Check sheet for the modelled part. Datum: model origin and axes. Units: mm. Face numbers are marked on the shaded views. A direction names the side the tool comes from. Give positions to 0.01 mm unless a question says otherwise; leave off trailing zeros. Loops run counter-clockwise (first coordinate to the right, second up) from the corner with the lowest first, then second, coordinate; pieces in that order, holes last. Notation, with made-up numbers: (8.25, 7.25) -> (20.25, 7.25) arc R17 cw to (20.25, 13.25) -> close; hole circle Ø3 at (85, -25.75). An arc over 180 degrees is marked (long way). Answer as CSV lines item,"result". Start each with the question number.
(1) Gauge pin test, flat end, axial feed: pin 1 Ø0.6 at (x, z) = (15, 1) entering from -Y. Record the tip position at first contact, or that the pin passes through.
(2) Material ranges on line 1 (Y direction, x = 13.45, z = 1.35) (3 decimals); line 2 (X direction, y = 2.5, z = 1.25); line 3 (Y direction, x = 2, z = 1) (3 decimals), recorded low to high. Write a range as from..to.
(3) Section check B-B on z = 1.45. Enter the section's corners in (x, y) (3 decimals), plus the area to 3 significant figures.
(4) Section check C-C on x = 1.5. Enter the section's corners in (y, z) (1 decimal).
(5) Release check for a two-part mould opening along Y. For the marked faces 4, 5, 6 and 7 record: pulls with the +Y half, pulls with the -Y half, needs draft (parallel to the pull), parting line crosses it, or undercut.
(6) Access from +Z, -Z, +X, -X, +Y, -Y to the whole of each face (thin tool, end or side, straight path). Record for the marked faces 1, 2 and 3.
(7) Section check A-A on x = 13.45. Enter the section's corners in (y, z) (3 decimals), plus the area to 3 significant figures.
from build123d import *

# Parameters (mm, degrees)
SKETCH2_R           = 0.95
BOSS_EXTRUDE1_DEPTH = 4
SKETCH3_W           = 16.2
SKETCH3_H           = 19.455
CUT_EXTRUDE1_DEPTH  = 2


with BuildPart() as part:
    # Sketch2 → Boss-Extrude1 (new body)
    with BuildSketch(Plane.XY):
        with BuildLine():
            Line((0, 7), (0, 12.455))
            Line((0, 12.455), (4, 12.455))
            Line((4, 12.455), (4, 14.455))
            Line((4, 14.455), (0, 14.455))
            Line((0, 14.455), (0, 17.455))
            ThreePointArc((0, 17.455), (0.585786438, 18.869213562), (2, 19.455))
            Line((2, 19.455), (14.2, 19.455))
            ThreePointArc((14.2, 19.455), (15.614213562, 18.869213562), (16.2, 17.455))
            Line((16.2, 17.455), (16.2, 14.455))
            Line((16.2, 14.455), (12.2, 14.455))
            Line((12.2, 14.455), (12.2, 12.455))
            Line((12.2, 12.455), (16.2, 12.455))
            Line((16.2, 12.455), (16.2, 7))
            Line((16.2, 7), (12.2, 7))
            Line((12.2, 7), (12.2, 5))
            Line((12.2, 5), (16.2, 5))
            Line((16.2, 5), (16.2, 2))
            ThreePointArc((16.2, 2), (15.614213562, 0.585786438), (14.2, 0))
            Line((14.2, 0), (2, 0))
            ThreePointArc((2, 0), (0.585786438, 0.585786438), (0, 2))
            Line((0, 2), (0, 5))
            Line((0, 5), (4, 5))
            Line((4, 5), (4, 7))
            Line((4, 7), (0, 7))
        make_face()
        with Locations((13.45, 2.5)):
            Circle(SKETCH2_R, mode=Mode.SUBTRACT)
        with Locations((2.75, 16.955)):
            Circle(SKETCH2_R, mode=Mode.SUBTRACT)
        with Locations((2.75, 2.5)):
            Circle(SKETCH2_R, mode=Mode.SUBTRACT)
        with Locations((13.45, 16.955)):
            Circle(SKETCH2_R, mode=Mode.SUBTRACT)
    extrude(amount=BOSS_EXTRUDE1_DEPTH)

    # Sketch3 → Cut-Extrude1 (cut)
    with BuildSketch(Plane.XY.offset(4)):
        with Locations((8.1, 9.7275)):
            Rectangle(SKETCH3_W, SKETCH3_H)
    extrude(amount=-CUT_EXTRUDE1_DEPTH, mode=Mode.SUBTRACT)


solid = part.part
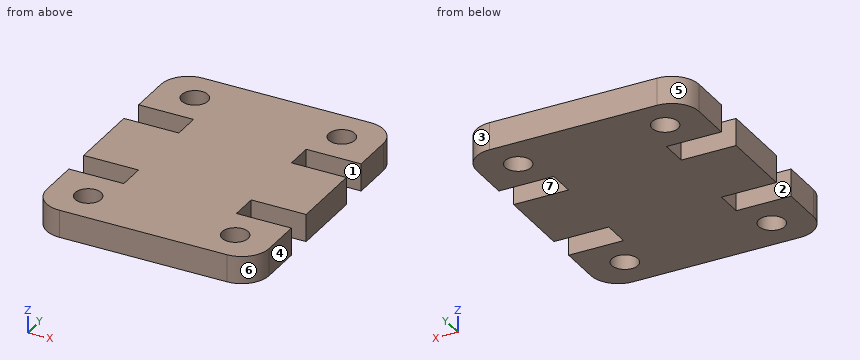
Working result:
1,pin 1,"stops at y = 0.06"
2,line 1,"y = 0..1.55, 3.45..5, 7..12.455, 14.455..16.005, 17.905..19.455"
2,line 2,"x = 0..1.8, 3.7..12.5, 14.4..16.2"
2,line 3,"y = 0..1.917, 3.083..5, 7..12.455, 14.455..16.372, 17.538..19.455"
3,outline,"(0, 2) arc R2 ccw to (2, 0) -> (14.2, 0) arc R2 ccw to (16.2, 2) -> (16.2, 5) -> (12.2, 5) -> (12.2, 7) -> (16.2, 7) -> (16.2, 12.455) -> (12.2, 12.455) -> (12.2, 14.455) -> (16.2, 14.455) -> (16.2, 17.455) arc R2 ccw to (14.2, 19.455) -> (2, 19.455) arc R2 ccw to (0, 17.455) -> (0, 14.455) -> (4, 14.455) -> (4, 12.455) -> (0, 12.455) -> (0, 7) -> (4, 7) -> (4, 5) -> (0, 5) -> close; hole circle Ø1.9 at (2.75, 2.5); hole circle Ø1.9 at (2.75, 16.955); hole circle Ø1.9 at (13.45, 2.5); hole circle Ø1.9 at (13.45, 16.955)"
3,area,"268 mm^2"
4,outline,"(0.1, 0) -> (5, 0) -> (5, 2) -> (0.1, 2) -> close; (7, 0) -> (12.5, 0) -> (12.5, 2) -> (7, 2) -> close; (14.5, 0) -> (19.4, 0) -> (19.4, 2) -> (14.5, 2) -> close"
5,face 4,"needs draft"
5,face 5,"pulls with the +Y half"
5,face 6,"pulls with the -Y half"
5,face 7,"undercut"
6,face 1,"+Z, -Z, +X"
6,face 2,"+Z, -Z, -X"
6,face 3,"+Z, -Z, +X, +Y"
7,outline,"(0, 0) -> (1.55, 0) -> (1.55, 2) -> (0, 2) -> close; (3.45, 0) -> (5, 0) -> (5, 2) -> (3.45, 2) -> close; (7, 0) -> (12.455, 0) -> (12.455, 2) -> (7, 2) -> close; (14.455, 0) -> (16.005, 0) -> (16.005, 2) -> (14.455, 2) -> close; (17.905, 0) -> (19.455, 0) -> (19.455, 2) -> (17.905, 2) -> close"
7,area,"23.3 mm^2"
